Autodesk Inventor part; units mm, degrees
ref_plane "YZ Plane" through (0, 0, 0) normal (1, 0, 0) x (0, 1, 0)
ref_plane "XZ Plane" through (0, 0, 0) normal (0, 1, 0) x (-1, 0, 0)
ref_plane "XY Plane" through (0, 0, 0) normal (0, 0, 1) x (1, 0, 0)
sketch "Esquisse2" plane through (0, 0, 0) normal (1, 0, 0) x (0, 1, 0)
  line L0 (-23.32, 215.2) -> (-23.32, 200.2)
  line L1 (-23.32, 200.2) -> (20.32, 200.2)
  spline S0 degree 4 poles (20.32, 200.2) (20.32, 180.2) (33.0773, 176.0923) (50, 129.3731) (47.5, 42) (47.5, 32) knots 1 1 1 1 1 2 3 3 3 3 3
  line L2 (47.5, 32) -> (47.5, 0)
  line L3 (-23.32, 200.2) -> (-23.32, 0)
  line L4 (-23.32, 0) -> (47.5, 0)
  line L5 (-39.8184, 0) -> (75.6707, 0)
  point P0 (0, 0)
revolve "Révolution1" add sketch "Esquisse2" angle 360 about axis through (0, -10, 0) along (0, 1, 0)
sketch "Esquisse3" plane through (0, -23.32, 0) normal (0, -1, 0) x (1, 0, 0)
  circle A0 centre (-254.2, 0) radius 4
  circle A1 centre (254.2, 0) radius 4
  circle A2 centre (-20, -253.412) radius 4
  circle A3 centre (20, -253.412) radius 4
  circle A4 centre (-20, 253.412) radius 4
  circle A5 centre (20, 253.412) radius 4
  circle A6 centre (-22, 0) radius 2.5
  circle A7 centre (-11, 19.0526) radius 2.5
  circle A8 centre (11, 19.0526) radius 2.5
  circle A9 centre (22, 0) radius 2.5
  circle A10 centre (11, -19.0526) radius 2.5
  circle A11 centre (-11, -19.0526) radius 2.5
  line L0 (70.7107, 254.5584) -> (254.5584, 70.7107)
  arc A12 (254.5584, -70.7107) -> (254.5584, 70.7107) centre (183.8478, 0) ccw
  line L1 (254.5584, -70.7107) -> (70.7107, -254.5584)
  arc A13 (-70.7107, -254.5584) -> (70.7107, -254.5584) centre (0, -183.8478) ccw
  line L2 (-70.7107, -254.5584) -> (-254.5584, -70.7107)
  arc A14 (-254.5584, 70.7107) -> (-254.5584, -70.7107) centre (-183.8478, 0) ccw
  line L3 (-254.5584, 70.7107) -> (-70.7107, 254.5584)
  arc A15 (70.7107, 254.5584) -> (-70.7107, 254.5584) centre (0, 183.8478) ccw
extrude "Extrusion1" add sketch "Esquisse3" along normal blind 23
sketch "Esquisse6" plane through (0, 47.5, 0) normal (0, 1, 0) x (1, 0, 0)
  circle A0 centre (20, -253.412) radius 4
  circle A1 centre (-20, -253.412) radius 4
  circle A2 centre (20, 253.412) radius 4
  circle A3 centre (-20, 253.412) radius 4
  circle A4 centre (254.2, 0) radius 4
  circle A5 centre (-254.2, 0) radius 4
  circle A6 centre (-11, 19.0526) radius 2.5
  circle A7 centre (11, 19.0526) radius 2.5
  circle A8 centre (22, 0) radius 2.5
  circle A9 centre (11, -19.0526) radius 2.5
  circle A10 centre (-11, -19.0526) radius 2.5
  circle A11 centre (-22, 0) radius 2.5
  line L0 (254.5584, -70.7107) -> (70.7107, -254.5584)
  arc A12 (-70.7107, -254.5584) -> (70.7107, -254.5584) centre (0, -183.8478) ccw
  line L1 (-70.7107, -254.5584) -> (-254.5584, -70.7107)
  arc A13 (-254.5584, 70.7107) -> (-254.5584, -70.7107) centre (-183.8478, 0) ccw
  line L2 (-254.5584, 70.7107) -> (-70.7107, 254.5584)
  arc A14 (70.7107, 254.5584) -> (-70.7107, 254.5584) centre (0, 183.8478) ccw
  line L3 (70.7107, 254.5584) -> (254.5584, 70.7107)
  arc A15 (254.5584, -70.7107) -> (254.5584, 70.7107) centre (183.8478, 0) ccw
  point P0 (0, -32)
extrude "Extrusion3" cut sketch "Esquisse6" against normal blind 35 contours A6 | A7 | A8 | A9 | A10 | A11
properties part number "wheel_rim_mold_C"
Geometry check sheet. Reference: the model listing, model coordinates, mm. A direction names the side the tool comes from. Coordinates: 2 decimals unless noted, no trailing zeros. Write each loop counter-clockwise with the first axis right and the second up, starting at its lowest first coordinate (ties: lowest second). Pieces come first, ordered by that corner, then holes. Notation, with made-up numbers: M 6,52.5 L 30,52.5 A31 cw 30,85.5 Z; hole C -33.75,13.25 d3. An arc over 180 degrees is marked long. One line per item, written item: value. Start each with the question number.
(1) Tool access check on faces 1 (the face through (168.809, -1.195, 107.626)), 2 (the face through (283.84, -34.66, 1.1)). Record the directions out of +Z, -Z, +X, -X, +Y, -Y that give a thin tool (end or side, any length) a straight path to the whole face; none if there is none.
(2) Scan lines: line 1 along Z through (x, y) = (11, 24.5); line 2 along Y through (x, z) = (-20.5, -47.5); line 3 along X through (y, z) = (13, 20). Record each from-to range of solid material in increasing order. Write a range as [from, to].
(3) Sectioned sample at A-A, the plane y = 4. Enter the section's corners in (x, z), and give its area (3 significant figures).
(4) Sectioned sample at C-C, the plane z = -208. Enter the section's corners in (x, y), and give its area (3 significant figures).
(5) Sectioned sample at B-B, the plane x = 241.5. Enter the section's corners in (y, z), and give its area (3 significant figures).
(6) Depth check by flat-ended pin: pin 1 (4 mm diameter, centred on x = -41, y = -33, fed in from -Z); pin 2 (6 mm diameter, centred on y = -2, z = 115.5, fed in from -X); pin 3 (12 mm diameter, centred on x = -62.5, z = 33, fed in from +Y). Enter the tip coordinate at first touch or a pass-through.
Filled sheet:
1. face 1: +Y
1. face 2: +X, +Y, -Y
2. line 1: [-179.8, -21.55], [-16.55, 16.55], [21.55, 179.8]
2. line 2: [-46.32, 47.62]
2. line 3: [-199.2, -13.31], [-8.69, 8.69], [13.31, 199.2]
3. outline: C 0,0 d400.4
3. area: 126,000 mm²
4. outline: M -117.27,-46.32 L 117.27,-46.32 L 117.27,-23.32 L -117.27,-23.32 Z
4. area: 5,390 mm²
5. outline: M -46.32,-83.77 L -23.32,-83.77 L -23.32,83.77 L -46.32,83.77 Z
5. area: 3,850 mm²
6. pin 1: z = -275.93
6. pin 2: x = -165.6
6. pin 3: y = 47.49
